Autodesk Inventor part; units mm, degrees
ref_plane "YZ Plane" through (0, 0, 0) normal (1, 0, 0) x (0, 1, 0)
ref_plane "XZ Plane" through (0, 0, 0) normal (0, 1, 0) x (-1, 0, 0)
ref_plane "XY Plane" through (0, 0, 0) normal (0, 0, 1) x (1, 0, 0)
sketch "スケッチ1" plane through (0, 0, 0) normal (0, 0, 1) x (1, 0, 0)
  line L0 (0, 0) -> (100, 0)
  line L1 (100, 0) -> (100, 100)
  line L2 (100, 100) -> (0, 100)
  line L3 (0, 100) -> (0, 0)
  dimension "d0" = 100
  dimension "d1" = 100
extrude "押し出し1" add sketch "スケッチ1" along normal blind 5
sketch "スケッチ2" plane through (0, 0, 0) normal (0, -1, 0) x (1, 0, 0)
  line L0 (100, 5) -> (0, 5)
  line L1 (50, 5) -> (50, 0) construction
  line L2 (100, 0) -> (0, 0)
  line L3 (85, 0) -> (15, 0)
  line L4 (15, 0) -> (15, 2.5)
  line L5 (15, 2.5) -> (85, 2.5)
  line L6 (85, 2.5) -> (85, 0)
  point P0 (15, 0)
  dimension "d4" = 70
  dimension "d5" = 2.5
extrude "押し出し2" add sketch "スケッチ2" along normal blind 10
sketch "スケッチ3" plane through (0, 0, 5) normal (0, 0, 1) x (1, 0, 0)
  line L0 (100, 100) -> (0, 100)
  line L1 (50, 100) -> (50, 0) construction
  line L2 (15, 0) -> (85, 0)
  point P0 (0, 0)
  point P1 (50, 20)
  dimension "d15" = 20
hole "穴1" at (50, 20, 5) direction (0, 0, -1) diameter 7 end through all
sketch "スケッチ5" plane through (0, 100, 0) normal (0, 1, 0) x (1, 0, 0)
  line L0 (53.5, -5) -> (46.5, -5)
  line L1 (50, -5) -> (50, 0) construction
  line L2 (46.5, 0) -> (53.5, 0)
  line L3 (100, 0) -> (0, 0)
  line L4 (15, 0) -> (85, 0)
  line L5 (85, 0) -> (85, -2.5)
  line L6 (85, -2.5) -> (15, -2.5)
  line L7 (15, -2.5) -> (15, 0)
  dimension "d25" = 2.5
  dimension "d26" = 70
extrude "押し出し3" add sketch "スケッチ5" along normal blind 2
properties part number "body_right"
Could you check a few things on this model? Use its own coordinates, in mm. A direction names the side the tool comes from. Give positions to 0.01 mm unless a question says otherwise; leave off trailing zeros. Order: outer loops, then holes, each group sorted by start corner. A loop starts at its lowest first (then second) coordinate and runs counter-clockwise, first axis right, second up. Notation, with made-up numbers: (-5.75, -8) -> (36.25, -8) arc R20 ccw to (36.25, 14) -> close; hole circle Ø10 at (87, 34). An arc over 180 degrees is marked (long way). Answer in a Markdown table with one row per item. Add a question column.
Item 1: I'm going to push flat-ended pins straight in: P1, Ø1.6, axis at x = 54, y = 101, coming from the +Z side; P2, Ø1.2, axis at y = -7, z = 2, coming from the +X side; P3, Ø1.6, axis at y = 101.5, z = 1, coming from the -X side. Where does each tip first touch, or does it pass through?
Item 2: We'd pull the mould along Y, two halves only. Please class faces 1 (the flat face through (85, -5, 1)), 2 (the cylindrical face through (46.53, 20.46, 2.46)), 3 (the flat face through (50, 102, 1)), 4 (the flat face through (50, -10, 1)): pulls with the +Y half, pulls with the -Y half, needs draft (parallel to the pull), parting line crosses it, or undercut.
Item 3: For faces 5 (the flat face through (0, 51, 2)), 6 (the flat face through (50, -5, 2.5)), 7 (the flat face through (15, -5, 1)), which set-ups out of +Z, -Z, +X, -X, +Y, -Y let a thin tool reach every point of the face, with its end or its side?
Item 4: Imagine slicing it at A-A (x = 50). List the corners of the cut face in (y, z) for me.
Item 5: Please list where these lines run through material, in increasing order: probe 1 along X at (y, z) = (20, 2.1); probe 2 along Y at (x, z) = (50, 1.6); probe 3 along Y at (x, z) = (50, 2.8).
Item 6: Imagine slicing it at C-C (x = 91.5). List the corners of the cut face in (y, z) for me, and give its area (3 significant figures).
Item 7: Imagine slicing it at B-B (y = 20). List the corners of the cut face in (x, z) for me, and give its area (3 significant figures).
Result:
| question | item | result |
|---|---|---|
| 1 | P1 | z = 2.5 |
| 1 | P2 | x = 85 |
| 1 | P3 | x = 15 |
| 2 | face 1 | needs draft |
| 2 | face 2 | undercut |
| 2 | face 3 | pulls with the +Y half |
| 2 | face 4 | pulls with the -Y half |
| 3 | face 5 | +Z, -Z, -X, +Y, -Y |
| 3 | face 6 | +Z, +X, -X, -Y |
| 3 | face 7 | +Z, -Z, -X, -Y |
| 4 | outline | (-10, 0) -> (16.5, 0) -> (16.5, 5) -> (0, 5) -> (0, 2.5) -> (-10, 2.5) -> close; (23.5, 0) -> (102, 0) -> (102, 2.5) -> (100, 2.5) -> (100, 5) -> (23.5, 5) -> close |
| 5 | probe 1 | 0 to 46.5, 53.5 to 100 |
| 5 | probe 2 | -10 to 16.5, 23.5 to 102 |
| 5 | probe 3 | 0 to 16.5, 23.5 to 100 |
| 6 | outline | (0, 0) -> (100, 0) -> (100, 5) -> (0, 5) -> close |
| 6 | area | 500 mm2 |
| 7 | outline | (0, 0) -> (46.5, 0) -> (46.5, 5) -> (0, 5) -> close; (53.5, 0) -> (100, 0) -> (100, 5) -> (53.5, 5) -> close |
| 7 | area | 465 mm2 |
